Part model, mm, in its own coordinate system. A direction names the side the tool comes from. Give positions to 0.01 mm unless a question says otherwise; leave off trailing zeros. Write each loop counter-clockwise with the first axis right and the second up, starting at its lowest first coordinate (ties: lowest second). Pieces come first, ordered by that corner, then holes.
from build123d import *

# Parameters (mm, degrees)
SKETCH1_W           = 5
SKETCH1_H           = 5
BOSS_EXTRUDE1_DEPTH = 5
CUT_EXTRUDE1_DEPTH  = 2
CUT_EXTRUDE2_DEPTH  = 1
SKETCH4_W           = 3
SKETCH4_H           = 2
CUT_EXTRUDE3_DEPTH  = 3
SKETCH5_W           = 2
SKETCH5_H           = 2
CUT_EXTRUDE4_DEPTH  = 1
CUT_EXTRUDE5_DEPTH  = 1
CUT_EXTRUDE6_DEPTH  = 2
CUT_EXTRUDE7_DEPTH  = 1
CUT_EXTRUDE8_DEPTH  = 3
CUT_EXTRUDE9_DEPTH  = 3


with BuildPart() as part:
    # Sketch1 → Boss-Extrude1 (new body)
    with BuildSketch(Plane.XY):
        Rectangle(SKETCH1_W, SKETCH1_H)
    extrude(amount=BOSS_EXTRUDE1_DEPTH)

    # Sketch2 → Cut-Extrude1 (cut)
    with BuildSketch(Plane(origin=(0, 2.5, 0), x_dir=(1, 0, 0), z_dir=(0, 1, 0))):
        Polygon((-2.5, -5), (-0.5, -5), (-0.5, -2), (-1.5, -2), (-1.5, -4), (-2.5, -4), align=None)
    extrude(amount=-CUT_EXTRUDE1_DEPTH, mode=Mode.SUBTRACT)

    # Sketch3 → Cut-Extrude2 (cut)
    with BuildSketch(Plane.ZY.offset(2.5)):
        Polygon((4, 0.5), (2, 2.5), (4, 2.5), align=None)
    extrude(amount=-CUT_EXTRUDE2_DEPTH, mode=Mode.SUBTRACT)

    # Sketch4 → Cut-Extrude3 (cut)
    with BuildSketch(Plane.XY.offset(5)):
        with Locations((1, 1.5)):
            Rectangle(SKETCH4_W, SKETCH4_H)
    extrude(amount=-CUT_EXTRUDE3_DEPTH, mode=Mode.SUBTRACT)

    # Sketch5 → Cut-Extrude4 (cut)
    with BuildSketch(Plane.XY.offset(2)):
        with Locations((1.5, 1.5)):
            Rectangle(SKETCH5_W, SKETCH5_H)
    extrude(amount=-CUT_EXTRUDE4_DEPTH, mode=Mode.SUBTRACT)

    # Sketch6 → Cut-Extrude5 (cut)
    with BuildSketch(Plane.XY.offset(1)):
        Polygon((2.5, 0.5), (0.5, 2.5), (2.5, 2.5), align=None)
    extrude(amount=-CUT_EXTRUDE5_DEPTH, mode=Mode.SUBTRACT)

    # Sketch7 → Cut-Extrude6 (cut)
    with BuildSketch(Plane(origin=(0, 0.5, 0), x_dir=(1, 0, 0), z_dir=(0, 1, 0))):
        Polygon((2.5, -5), (2.5, -3), (1.5, -3), (-0.5, -5), align=None)
    extrude(amount=-CUT_EXTRUDE6_DEPTH, mode=Mode.SUBTRACT)

    # Sketch8 → Cut-Extrude7 (cut)
    with BuildSketch(Plane(origin=(2.5, 0, 0), x_dir=(0, 0, -1), z_dir=(1, 0, 0))):
        Polygon((-3, -1.5), (-2, 0.5), (-3, 0.5), align=None)
    extrude(amount=-CUT_EXTRUDE7_DEPTH, mode=Mode.SUBTRACT)

    # Sketch9 → Cut-Extrude8 (cut)
    with BuildSketch(Plane(origin=(2.5, 0, 0), x_dir=(0, 0, -1), z_dir=(1, 0, 0))):
        Polygon((-5, -1.5), (-4, 0.5), (-5, 0.5), align=None)
    extrude(amount=-CUT_EXTRUDE8_DEPTH, mode=Mode.SUBTRACT)

    # Sketch11 → Cut-Extrude9 (cut)
    with BuildSketch(Plane(origin=(1.666666667, 0.833333333, 1.666666667), x_dir=(-0.745355992, 0.298142397, 0.596284794), z_dir=(-0.666666667, -0.333333333, -0.666666667))):
        Polygon((2.906888371, -1.341640786), (0.223606798, -0.447213595), (0.223606798, -2.683281573), (2.906888371, -3.577708764), align=None)
    extrude(amount=-CUT_EXTRUDE9_DEPTH, mode=Mode.SUBTRACT)


solid = part.part
1) Saw through at D-D (y = -0.6). Write the cut outline in (x, z).
Check result:
outline: (-2.5, 0) - (2.5, 0) - (2.5, 2.55) - (1.5, 2.55) - (-0.5, 4.55) - (-0.5, 5) - (-2.5, 5) - close
2) Flat gauge pins, fed straight in: P1, Ø3, axis at x = 1.5, y = 0.5, coming from the +Z side; P2, Ø1.5, axis at x = 0.5, z = 3, coming from the +Y side; P3, Ø1.6, axis at x = 1.5, y = 1, coming from the +Z side. Where does each tip first touch, or does it go through?
Check result:
P1: stops at z = 3.68
P2: stops at y = 0.5
P3: stops at z = 2.62
3) Saw through at B-B (x = 0.85). Write the cut outline in (y, z).
Check result:
outline: (-2.5, 0) - (2.15, 0) - (2.15, 1) - (0.5, 1) - (0.5, 2.65) - (-1.5, 3.65) - (-1.5, 5) - (-2.5, 5) - close
4) Saw through at A-A (y = 1.75). Write the cut outline in (x, z), and give its area (3 significant figures).
Check result:
outline: (-2.5, 0) - (1.25, 0) - (1.25, 1) - (0.5, 1) - (0.5, 2) - (-1.5, 2) - (-1.5, 2.75) - (-2.5, 2.75) - close
area: 7.50 mm2
5) 3-axis set-ups, long thin cutter, end or side, ignore diameter. For faces 1 (the flat face through (-1, 2.5, 1)), 2 (the flat face through (-1.5, 1, 3)): which of +Z, -Z, +X, -X, +Y, -Y reach the whole face in a straight line?
Check result:
face 1: +Z, -Z, +X, -X, +Y
face 2: +Z, +X, +Y
6) Drill centre lines: L1, parallel to Y at x = -0.2, z = 2.85; L2, parallel to Y at x = 0.9, z = 3.9; L3, parallel to Z at x = -1.9, y = 1.5. Where is each one in solid material? Low to high.
Check result:
L1: y = -2.5 to 0.5
L2: y = -2.5 to -1.5
L3: z = 0 to 3
7) Saw through at C-C (z = 4.65). Write the cut outline in (x, y), and give its area (3 significant figures).
Check result:
outline: (-2.5, -2.5) - (2.5, -2.5) - (2.5, -1.5) - (-0.15, -1.5) - (-0.5, -0.8) - (-0.5, 0.5) - (-2.5, 0.5) - close
area: 9.12 mm2
